Verification items for the finished model (mm, model axes). Round coordinates to 2 decimals unless told otherwise and drop trailing zeros. Order: outer loops, then holes, each group sorted by start corner. A loop starts at its lowest first (then second) coordinate and runs counter-clockwise, first axis right, second up. Notation, with made-up numbers: M 60.5,84 L 118.5,84 A34 ccw 118.5,122 Z; hole C 8,56.25 d9. An arc over 180 degrees is marked long. Use CSV: the item, a comma, the result in double quotes. Start each with the question number.
Q1. Sectioned sample at A-A (x = 0). Enter the section's corners in (y, z), and give its area (3 significant figures).
Q2. Sectioned sample at B-B (z = 2.1). Enter the section's corners in (x, y).
Q3. Mould release check, pull along X, two halves, no side actions. Record for faces 1 (the face through (26.67, -1, 2)), 2 (the face through (-24.33, 49.86, 2.22)), 3 (the face through (-0.92, -50.7, 2.22)): +X half, -X half, draft (parallel to the pull), parting line (faces both ways), or undercut.
Q4. Scan lines: line 1 (Y direction, x = 0, z = 2.05); line 2 (Y direction, x = 19, z = 3.1); line 3 (X direction, y = -48, z = 1.35). Record each from-to range of solid material in increasing order.
```python
from build123d import *

# Parameters (mm, degrees)
F0_R     = 4.220901
F1_DEPTH = 5
F2_R     = 0.5


with BuildPart() as f1:
    # F0 (on Top) → F1 (new body)
    with BuildSketch(Plane.XY):
        with BuildLine():
            ThreePointArc((26.67, 44.302669), (24.395001, 49.795001), (18.902669, 52.07))
            Line((18.902669, 52.07), (-18.902669, 52.07))
            ThreePointArc((-18.902669, 52.07), (-24.395001, 49.795001), (-26.67, 44.302669))
            Line((-26.67, 44.302669), (-26.67, -44.302669))
            ThreePointArc((-26.67, -44.302669), (-24.395001, -49.795001), (-18.902669, -52.07))
            Line((-18.902669, -52.07), (18.902669, -52.07))
            ThreePointArc((18.902669, -52.07), (24.395001, -49.795001), (26.67, -44.302669))
            Line((26.67, -44.302669), (26.67, 44.302669))
        make_face()
        with Locations((0, -46.580885)):
            Circle(F0_R, mode=Mode.SUBTRACT)
    extrude(amount=F1_DEPTH)

    # F2
    f2_edges = [f1.edges().sort_by_distance(p)[0] for p in [
        (26.67, 0, 5),
        (24.395001, 49.795001, 5),
        (0, 52.07, 5),
        (-24.395001, 49.795001, 5),
        (-26.67, 0, 5),
        (-24.395001, -49.795001, 5),
        (0, -52.07, 5),
        (24.395001, -49.795001, 5),
        (-4.220901, -46.580885, 5),
    ]]
    fillet(f2_edges, radius=F2_R)


solid = f1.part
```
Verdict:
1,outline,"M -52.07,0 L -50.8,0 L -50.8,4.5 A0.5 ccw -51.3,5 L -51.57,5 A0.5 ccw -52.07,4.5 Z; M -42.36,0 L 52.07,0 L 52.07,4.5 A0.5 ccw 51.57,5 L -41.86,5 A0.5 ccw -42.36,4.5 Z"
1,area,"478 mm²"
2,outline,"M -26.67,-44.3 A7.77 ccw -18.9,-52.07 L 18.9,-52.07 A7.77 ccw 26.67,-44.3 L 26.67,44.3 A7.77 ccw 18.9,52.07 L -18.9,52.07 A7.77 ccw -26.67,44.3 Z; hole C 0,-46.58 d8.44"
3,face 1,"+X half"
3,face 2,"-X half"
3,face 3,"undercut"
4,line 1,"y = -52.07 to -50.8, -42.36 to 52.07"
4,line 2,"y = -52.07 to 52.07"
4,line 3,"x = -25.73 to -3.98, 3.98 to 25.73"
